from build123d import *

# Parameters (mm, degrees)
BOSS_EXTRUDE2_DEPTH = 30
SKETCH3_R           = 1.5
CUT_EXTRUDE1_DEPTH  = 6
SKETCH4_R           = 2
CUT_EXTRUDE2_DEPTH  = 6


with BuildPart() as part:
    # Sketch1 → Boss-Extrude2 (new body)
    with BuildSketch(Plane(origin=(0, 0, 0), x_dir=(1, 0, 0), z_dir=(0, 1, 0))):
        with BuildLine():
            Line((-4.850712501, 19.402850003), (-7.276068751, 29.104275004))
            ThreePointArc((-7.276068751, 29.104275004), (0, 30), (7.276068751, 29.104275004))
            Line((7.276068751, 29.104275004), (4.850712501, 19.402850003))
            ThreePointArc((4.850712501, 19.402850003), (0, 20), (-4.850712501, 19.402850003))
        make_face()
    extrude(amount=BOSS_EXTRUDE2_DEPTH)

    # Sketch3 → Cut-Extrude1 (cut)
    with BuildSketch(Plane.XZ):
        with Locations(Location((0, -25.024693025, 0), (0, 0, 270))):
            Circle(SKETCH3_R)
    extrude(amount=-CUT_EXTRUDE1_DEPTH, mode=Mode.SUBTRACT)

    # Sketch4 → Cut-Extrude2 (cut)
    with BuildSketch(Plane(origin=(0, 30, 0), x_dir=(1, 0, 0), z_dir=(0, 1, 0))):
        with Locations(Location((0, 23, 0), (0, 0, 270))):
            Circle(SKETCH4_R)
    extrude(amount=-CUT_EXTRUDE2_DEPTH, mode=Mode.SUBTRACT)


solid = part.part
The model under review builds one solid part; all positions refer to its coordinate system, in mm. A direction names the side the tool comes from. Round coordinates to 2 decimals unless told otherwise and drop trailing zeros. Order: outer loops, then holes, each group sorted by start corner. A loop starts at its lowest first (then second) coordinate and runs counter-clockwise, first axis right, second up. Notation, with made-up numbers: (20, 68.5) -> (33, 68.5) arc R21 cw to (33, 84.5) -> close; hole circle Ø9 at (47.5, 49.25). An arc over 180 degrees is marked (long way). Use CSV: the item, a comma, the result in double quotes. Start each with the question number.
(1) Consider section B-B on z = -23. Write out the cut boundary in (x, y).
(2) Insertion check: pin 1 (2 mm diameter, centred on x = 0, z = -23, fed in from +Y); pin 2 (2 mm diameter, centred on x = -4.5, y = 3, fed in from -Z); pin 3 (0.9 mm diameter, centred on x = 0.5, z = -25, fed in from -Y). Each pin has a flat end and moves straight along its axis. Give the tip position at first contact, or say it passes through.
(3) Consider section D-D on z = -21.75. Write out the cut boundary in (x, y), and give its area (3 significant figures).
(4) Wall thickness on probe 1 along X at (y, z) = (26.15, -23); probe 2 along X at (y, z) = (3.5, -26); probe 3 along Y at (x, z) = (1.5, -22.5): over which ranges is each line inside the solid? List them lowest first. Write a range as from..to.
(5) Consider section C-C on y = 26.75. Write out the cut boundary in (x, z), and give its area (3 significant figures).
(6) Mouldability with a two-part tool opening along Z and no side actions: class faces 4 (the face through (0, 30, -26)), 5 (the face through (-6, 15, -24)), 6 (the face through (-1.2, 27, -24.6)) as pulls with the +Z half, pulls with the -Z half, needs draft (parallel to the pull), parting line crosses it, or undercut.
(7) Consider section A-A on y = 2.75. Write out the cut boundary in (x, z).
(8) Tool access review of faces 1 (the face through (0, 6, -25)), 2 (the face through (0, 24, -23)), 3 (the face through (6, 15, -24)): name each direction out of +Z, -Z, +X, -X, +Y, -Y from which nothing blocks a thin tool from reaching the whole face with its end or side.
Responses:
1,outline,"(-5.75, 0) -> (5.75, 0) -> (5.75, 30) -> (2, 30) -> (2, 24) -> (-2, 24) -> (-2, 30) -> (-5.75, 30) -> close"
2,pin 1,"y = 24"
2,pin 2,"z = -29.8"
2,pin 3,"y = 6"
3,outline,"(-5.44, 0) -> (5.44, 0) -> (5.44, 30) -> (1.56, 30) -> (1.56, 24) -> (-1.56, 24) -> (-1.56, 30) -> (-5.44, 30) -> close"
3,area,"308 mm²"
4,probe 1,"-5.75..-2, 2..5.75"
4,probe 2,"-6.5..-1.14, 1.14..6.5"
4,probe 3,"0..24"
5,outline,"(-7.28, -29.1) arc R30 ccw to (7.28, -29.1) -> (4.85, -19.4) arc R20 cw to (-4.85, -19.4) -> close; hole circle Ø4 at (0, -23)"
5,area,"110 mm²"
6,face 4,"needs draft"
6,face 5,"pulls with the +Z half"
6,face 6,"undercut"
7,outline,"(-7.28, -29.1) arc R30 ccw to (7.28, -29.1) -> (4.85, -19.4) arc R20 cw to (-4.85, -19.4) -> close; hole circle Ø3 at (0, -25.02)"
8,face 1,"-Y"
8,face 2,"+Y"
8,face 3,"+Z, +X, +Y, -Y"
